The listing builds one solid part. Answer for the finished solid, in the listing's coordinates (mm). A direction names the side the tool comes from. Round coordinates to 2 decimals unless told otherwise and drop trailing zeros. Write each loop counter-clockwise with the first axis right and the second up, starting at its lowest first coordinate (ties: lowest second). Pieces come first, ordered by that corner, then holes.
Item 1: Find section B-B on x = 26.5. Give the vertices of the cut face in (y, z).
Item 2: A tool of negligible diameter and unlimited length cuts with its end or side. For faces 4 (the face through (-5.699, -21.143, -0.021)), 5 (the face through (5, 23, 0)), 6 (the face through (-13, 0, -7.5)), 7 (the face through (21, -10, 3)), 8 (the face through (-9.76, -16.3, -2.49)), from which of +Z, -Z, +X, -X, +Y, -Y can it reach the whole face along a straight path? Write none if from no direction.
Item 3: For a pull along X with two mould halves and no side action, classify faces 1 (the face through (21, 12, 0)), 2 (the face through (40, 0, 0)), 3 (the face through (-7, 37, -2)) as +X half, -X half, draft (parallel to the pull), parting line (faces both ways), or undercut.
Item 4: Find the intervals of material crossed by probe 1 along X at (y, z) = (0, 0.2); probe 2 along X at (y, z) = (-21, -2.75); probe 3 along X at (y, z) = (27, 0.7), in increasing order.
Item 5: Find section A-A on z = -5.75. Give the vertices of the cut face in (x, y), then the cut area to 3 significant figures.
Item 6: Find section C-C on y = -22.5. Give the vertices of the cut face in (x, z).
Item 7: Each of these flat-tipped pins is pushed along its axis until it touches: pin 1 (14 mm diameter, centred on x = -7, y = -27, fed in from +Z); pin 2 (0.6 mm diameter, centred on x = 17.5, z = 2.5, fed in from -Y); pin 3 (2 mm diameter, centred on x = 22, z = -2.5, fed in from +Y). Where does it stop, or does it pass through?
```python
from build123d import *
from build123d.topology import SkipClean

# Parameters (mm, degrees)
ESQUISSE1_R                  = 9
ESQUISSE1_R_2                = 6
EXTRUSION1_DEPTH             = 3.5
ENL_V_MAT_EXTRU_1_DEPTH      = 2
ENL_V_START                  = -2
ESQUISSE4_R                  = 17
ENL_V_MAT_EXTRU_2_DEPTH      = 2
ESQUISSE6_W                  = 7.877170109
ESQUISSE6_H                  = 1.5
EXTRUSION4_DEPTH             = 6
R_P_TITION_CIRCULAIRE1_COUNT = 2
EXTRUSION5_START             = 3
EXTRUSION5_DEPTH             = 3
ENL_V_MAT_EXTRU_3_DEPTH      = 3
ESQUISSE10_R                 = 3.5
EXTRUSION6_DEPTH             = 3
ESQUISSE11_R                 = 1.5
ENL_V_MAT_EXTRU_4_DEPTH      = 57.938563382


with BuildPart() as part:
    # Esquisse1 → Extrusion1 (new, symmetric)
    with BuildSketch(Plane.XY):
        with BuildLine():
            Line((28, 12), (14.730919863, 12))
            ThreePointArc((14.730919863, 12), (10.360766525, 15.926534997), (5, 18.33030278))
            Line((5, 18.33030278), (5, 27))
            ThreePointArc((5, 27), (-7, 39), (-19, 27))
            Line((-19, 27), (-19, 6))
            Line((-19, 6), (-18.35969719, 4.890963001))
            ThreePointArc((-18.35969719, 4.890963001), (-19, 0), (-18.35969719, -4.890963001))
            Line((-18.35969719, -4.890963001), (-19, -6))
            Line((-19, -6), (-19, -27))
            ThreePointArc((-19, -27), (-7, -39), (5, -27))
            Line((5, -27), (5, -18.33030278))
            ThreePointArc((5, -18.33030278), (10.360766525, -15.926534997), (14.730919863, -12))
            Line((14.730919863, -12), (28, -12))
            ThreePointArc((28, -12), (40, 0), (28, 12))
        make_face()
        with Locations(Location((0, 0, 0), (0, 0, 127.669886964))):
            Circle(ESQUISSE1_R, mode=Mode.SUBTRACT)
        with Locations(Location((-7, -27, 0), (0, 0, 180))):
            Circle(ESQUISSE1_R_2, mode=Mode.SUBTRACT)
        with Locations((-7, 27)):
            Circle(ESQUISSE1_R_2, mode=Mode.SUBTRACT)
        with Locations((28, 0)):
            Circle(ESQUISSE1_R_2, mode=Mode.SUBTRACT)
    extrude(amount=EXTRUSION1_DEPTH, both=True)

    # Esquisse3 → Enlèv. mat.-Extru.1 (cut)
    with BuildSketch(Plane.XY.offset(3.5)):
        with BuildLine():
            Line((-16.200693523, -5.151458956), (-17, -6.535898385))
            Line((-17, -6.535898385), (-17, -27))
            ThreePointArc((-17, -27), (-7, -37), (3, -27))
            Line((3, -27), (3, -16.733200531))
            ThreePointArc((3, -16.733200531), (9.025274953, -14.406401772), (13.747727085, -10))
            Line((13.747727085, -10), (28, -10))
            ThreePointArc((28, -10), (38, 0), (28, 10))
            Line((28, 10), (13.747727085, 10))
            ThreePointArc((13.747727085, 10), (9.025274953, 14.406401772), (3, 16.733200531))
            Line((3, 16.733200531), (3, 27))
            ThreePointArc((3, 27), (-7, 37), (-17, 27))
            Line((-17, 27), (-17, 6.535898385))
            Line((-17, 6.535898385), (-16.200693523, 5.151458956))
            ThreePointArc((-16.200693523, 5.151458956), (-17, 0), (-16.200693523, -5.151458956))
        make_face()
    extrude(amount=-ENL_V_MAT_EXTRU_1_DEPTH, mode=Mode.SUBTRACT)

    # Esquisse4 → Enlèv. mat.-Extru.2 (cut)
    with BuildSketch(Plane(origin=(0, 0, -3.5), x_dir=(-1, 0, 0), z_dir=(0, 0, -1)).offset(ENL_V_START)):
        Circle(ESQUISSE4_R)
        with BuildLine():
            Line((17, 12), (17, 27))
            ThreePointArc((17, 27), (7, 37), (-3, 27))
            Line((-3, 27), (-3, 19.899748742))
            ThreePointArc((-3, 19.899748742), (-2.670820393, 19.158128893), (-1.9, 18.904761305))
            ThreePointArc((-1.9, 18.904761305), (7.635630986, 17.398193568), (15.2, 11.4))
            ThreePointArc((15.2, 11.4), (16.316227766, 11.051316702), (17, 12))
        make_face()
        with BuildLine():
            Line((-17.860571099, 10), (-28, 10))
            ThreePointArc((-28, 10), (-38, 0), (-28, -10))
            Line((-28, -10), (-17.860571099, -10))
            ThreePointArc((-17.860571099, -10), (-17.009101781, -9.524404424), (-16.967542545, -8.55))
            ThreePointArc((-16.967542545, -8.55), (-19, 0), (-16.967542545, 8.55))
            ThreePointArc((-16.967542545, 8.55), (-17.009101781, 9.524404424), (-17.860571099, 10))
        make_face()
        with BuildLine():
            Line((-3, -19.899748742), (-3, -27))
            ThreePointArc((-3, -27), (7, -37), (17, -27))
            Line((17, -27), (17, -12))
            ThreePointArc((17, -12), (16.316227766, -11.051316702), (15.2, -11.4))
            ThreePointArc((15.2, -11.4), (7.635630986, -17.398193568), (-1.9, -18.904761305))
            ThreePointArc((-1.9, -18.904761305), (-2.670820393, -19.158128893), (-3, -19.899748742))
        make_face()
    extrude(amount=ENL_V_MAT_EXTRU_2_DEPTH, mode=Mode.SUBTRACT)

    # Esquisse6 → Extrusion4 (add)
    with BuildSketch(Plane(origin=(0, 0, -1.5), x_dir=(-1, 0, 0), z_dir=(0, 0, -1))):
        with Locations((13.200835764, 0)):
            Rectangle(ESQUISSE6_W, ESQUISSE6_H)
    extrusion4 = extrude(amount=EXTRUSION4_DEPTH)

    # Répétition circulaire1: Extrusion4 ×2 about axis
    r_p_tition_circulaire1_axis = Axis((0, 0, 0), (0, 0, 1))
    for i in range(1, R_P_TITION_CIRCULAIRE1_COUNT):
        add(extrusion4.rotate(r_p_tition_circulaire1_axis, i * 360 / R_P_TITION_CIRCULAIRE1_COUNT))

    # Esquisse7 → Extrusion5 (add)
    with SkipClean():  # the faces are left unmerged after this step: merging them gives an invalid solid
        with BuildSketch(Plane(origin=(0, 0, -1.5), x_dir=(-1, 0, 0), z_dir=(0, 0, -1)).offset(EXTRUSION5_START)):
            with BuildLine():
                Line((5.5, 14), (5.5, 7.123903424))
                ThreePointArc((5.5, 7.123903424), (0, 9), (-5.5, 7.123903424))
                Line((-5.5, 7.123903424), (-5.5, 14))
                ThreePointArc((-5.5, 14), (0, 19.5), (5.5, 14))
            make_face()
            with BuildLine():
                Line((-5.5, -14), (-5.5, -7.123903424))
                ThreePointArc((-5.5, -7.123903424), (0, -9), (5.5, -7.123903424))
                Line((5.5, -7.123903424), (5.5, -14))
                ThreePointArc((5.5, -14), (0, -19.5), (-5.5, -14))
            make_face()
        extrude(amount=-EXTRUSION5_DEPTH)

    # Esquisse8 → Enlèv. mat.-Extru.3 (cut)
    with SkipClean():  # the faces are left unmerged after this step: merging them gives an invalid solid
        with BuildSketch(Plane.XY.offset(1.5)):
            with BuildLine():
                Line((3.5, 12.5), (3.5, -12.5))
                ThreePointArc((3.5, -12.5), (0, -16), (-3.5, -12.5))
                Line((-3.5, -12.5), (-3.5, 12.5))
                ThreePointArc((-3.5, 12.5), (0, 16), (3.5, 12.5))
            make_face()
        extrude(amount=-ENL_V_MAT_EXTRU_3_DEPTH, mode=Mode.SUBTRACT)

    # Esquisse10 → Extrusion6 (add)
    with SkipClean():  # the faces are left unmerged after this step: merging them gives an invalid solid
        with BuildSketch(Plane(origin=(0, 0, -4.5), x_dir=(-1, 0, 0), z_dir=(0, 0, -1))):
            with Locations(Location((0, 12.5, 0), (0, 0, 270))):
                Circle(ESQUISSE10_R)
            with Locations(Location((0, -12.5, 0), (0, 0, 89.999632483))):
                Circle(ESQUISSE10_R)
        extrude(amount=EXTRUSION6_DEPTH)

    # Esquisse11 → Enlèv. mat.-Extru.4 (cut, through all)
    with SkipClean():  # the faces are left unmerged after this step: merging them gives an invalid solid
        with BuildSketch(Plane(origin=(0, 0, -7.5), x_dir=(-1, 0, 0), z_dir=(0, 0, -1))):
            with Locations((0, -12.5)):
                Circle(ESQUISSE11_R)
            with Locations((0, 12.5)):
                Circle(ESQUISSE11_R)
        extrude(amount=-ENL_V_MAT_EXTRU_4_DEPTH, mode=Mode.SUBTRACT)


solid = part.part
```
Check values:
1. outline: (-12, -3.5) - (-10, -3.5) - (-10, -1.5) - (-5.81, -1.5) - (-5.81, 1.5) - (-10, 1.5) - (-10, 3.5) - (-12, 3.5) - close; (5.81, -1.5) - (10, -1.5) - (10, -3.5) - (12, -3.5) - (12, 3.5) - (10, 3.5) - (10, 1.5) - (5.81, 1.5) - close
2. face 4: +Z, -Z
2. face 5: +Z, -Z, +X, +Y
2. face 6: -Z, +X, -X, +Y, -Y
2. face 7: +Z
2. face 8: -Z
3. face 1: draft
3. face 2: +X half
3. face 3: undercut
4. probe 1: x = -19 to -9, 9 to 22, 34 to 40
4. probe 2: x = -19 to -17, 3 to 5
4. probe 3: x = -19 to -13, -1 to 5
5. outline: (-17.14, -0.75) - (-9.26, -0.75) - (-9.26, 0.75) - (-17.14, 0.75) - close; circle Ø7 at (0, -12.5); circle Ø7 at (0, 12.5); (9.26, -0.75) - (17.14, -0.75) - (17.14, 0.75) - (9.26, 0.75) - close; hole circle Ø3 at (0, -12.5); hole circle Ø3 at (0, 12.5)
5. area: 86.5 mm2
6. outline: (-19, -3.5) - (-17, -3.5) - (-17, -1.5) - (-10.97, -1.5) - (-10.97, 1.5) - (-17, 1.5) - (-17, 3.5) - (-19, 3.5) - close; (-3.03, -1.5) - (3, -1.5) - (3, -3.5) - (5, -3.5) - (5, 3.5) - (3, 3.5) - (3, 1.5) - (-3.03, 1.5) - close
7. pin 1: stops at z = 1.5
7. pin 2: stops at y = -12
7. pin 3: stops at y = 12
